from build123d import *

# Parameters (mm, degrees)
SKETCH_1_W       = 76
SKETCH_1_H       = 151
EXTRUDE_1_DEPTH  = 11
EXTRUDE_START    = -11
EXTRUDE_2_DEPTH  = 12
FILLET_1_R       = 5
WRAP_1_OUTLINE_R = 1
WRAP_1_DEPTH     = 0.01


# Read off the part's stored shape, not the designer's step: 包覆1
with BuildPart() as part:
    # 草图1 → 凸台-拉伸1 (new body)
    with BuildSketch(Plane(origin=(0, 0, 0), x_dir=(1, 0, 0), z_dir=(0, 1, 0))):
        Rectangle(SKETCH_1_W, SKETCH_1_H)
    extrude(amount=EXTRUDE_1_DEPTH)

    # 草图2 → 凸台-拉伸2 (add)
    with BuildSketch(Plane.XZ.offset(EXTRUDE_START)):
        with BuildLine():
            Line((10.145843496, 74.5), (24.854156504, 74.5))
            ThreePointArc((24.854156504, 74.5), (33.442564803, 70.942564803), (37, 62.354156504))
            Line((37, 62.354156504), (37, 47.354156504))
            ThreePointArc((37, 47.354156504), (34.331959922, 39.7585817), (27.5, 35.5))
            Line((27.5, 35.5), (7.5, 35.5))
            ThreePointArc((7.5, 35.5), (0.668040078, 39.7585817), (-2, 47.354156504))
            Line((-2, 47.354156504), (-2, 62.354156504))
            ThreePointArc((-2, 62.354156504), (1.557435197, 70.942564803), (10.145843496, 74.5))
        make_face()
    extrude(amount=EXTRUDE_2_DEPTH)

    # 圆角1
    fillet_1_edges = [part.edges().sort_by_distance(p)[0] for p in [
        (38, 5.5, 75.5),
        (-38, 5.5, 75.5),
        (-38, 5.5, -75.5),
        (38, 5.5, -75.5),
    ]]
    fillet(fillet_1_edges, radius=FILLET_1_R)

    # 包覆1 outline → 包覆1 (add)
    with BuildSketch(Plane.XZ):
        Circle(WRAP_1_OUTLINE_R)
    extrude(amount=WRAP_1_DEPTH)


solid = part.part
Geometry check sheet. Reference: the model listing, model coordinates, mm. A direction names the side the tool comes from. Round coordinates to 2 decimals unless told otherwise and drop trailing zeros. Order: outer loops, then holes, each group sorted by start corner. A loop starts at its lowest first (then second) coordinate and runs counter-clockwise, first axis right, second up. Notation, with made-up numbers: M 86.5,80.5 L 111.5,80.5 A33 ccw 111.5,108.5 Z; hole C 72.25,26 d3. An arc over 180 degrees is marked long. Answer in a Markdown table with one row per item. Add a question column.
Item 1: Depth check by flat-ended pin: pin 1 Ø0.5 at (x, y) = (15.5, -0.5) entering from -Z; pin 2 Ø8 at (x, z) = (-16, 39) entering from -Y; pin 3 Ø0.5 at (y, z) = (-0.5, 54) entering from +X. Enter the tip coordinate at first touch or a pass-through.
Item 2: Sectioned sample at B-B, the plane x = -13.5. Enter the section's corners in (y, z), plus the area to 3 significant figures.
Item 3: Sectioned sample at A-A, the plane z = -25. Enter the section's corners in (x, y), plus the area to 3 significant figures.
Item 4: Set-up check for faces 1 (the face through (0.74, -0.49, 39.67)), 2 (the face through (33.348, -0.493, 71.036)), 3 (the face through (1.464, -0.493, 70.848)): record each of +Z, -Z, +X, -X, +Y, -Y from which the full face is reachable in a straight line by a thin tool's end or side.
Item 5: Material ranges on L1, parallel to Y at x = -17.5, z = 32, recorded low to high. Write a range as [from, to].
Filled in:
| question | item | result |
|---|---|---|
| 1 | pin 1 | stops at z = 35.5 |
| 1 | pin 2 | stops at y = 0 |
| 1 | pin 3 | stops at x = 37 |
| 2 | outline | M 0,-75.5 L 11,-75.5 L 11,75.5 L 0,75.5 Z |
| 2 | area | 1,660 mm² |
| 3 | outline | M -38,0 L 38,0 L 38,11 L -38,11 Z |
| 3 | area | 836 mm² |
| 4 | face 1 | -Z, -X, -Y |
| 4 | face 2 | +Z, +X, -Y |
| 4 | face 3 | +Z, -X, -Y |
| 5 | L1 | y = [0, 11] |
